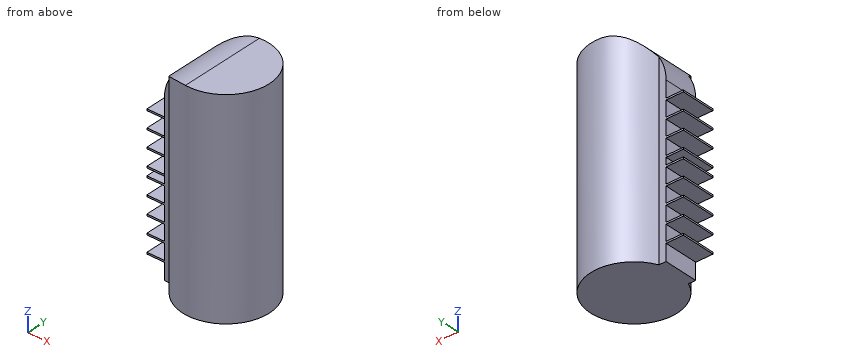
```python
from build123d import *

# Parameters (mm, degrees)
F1_DEPTH = 304.8
F2_R     = 63.5
F4_DEPTH = 25.4


with BuildPart() as f1:
    # F0 (on Top) → F1 (new body)
    with BuildSketch(Plane.XY):
        with BuildLine():
            Line((-68.801289, -25.4), (-58.198711, -25.4))
            ThreePointArc((-58.198711, -25.4), (63.5, 0), (-58.198711, 25.4))
            Line((-58.198711, 25.4), (-68.801289, 25.4))
            Line((-68.801289, 25.4), (-68.801289, -25.4))
        make_face()
    extrude(amount=F1_DEPTH)

    # F2
    f2_edges = [f1.edges().sort_by_distance(p)[0] for p in [
        (-68.801289, 0, 304.8),
    ]]
    fillet(f2_edges, radius=F2_R)

    # F3 (on face) → F4 (join)
    with BuildSketch(Plane(origin=(-68.801289, 0, 0), x_dir=(0, -1, 0), z_dir=(-1, 0, 0))):
        Polygon((-0.093374, 215.9), (-0.093374, 217.17), (-25.4, 217.17), (-25.4, 214.63), (-0.093374, 214.63), align=None)
        Polygon((25.213252, 217.17), (-0.093374, 217.17), (-0.093374, 215.9), (-0.093374, 214.63), (25.213252, 214.63), align=None)
        Polygon((-0.093374, 190.5), (-0.093374, 189.23), (25.213252, 189.23), (25.213252, 191.77), (-0.093374, 191.77), align=None)
        Polygon((-25.4, 191.77), (-25.4, 189.23), (-0.093374, 189.23), (-0.093374, 190.5), (-0.093374, 191.77), align=None)
        Polygon((-25.4, 166.37), (-25.4, 163.83), (-0.093374, 163.83), (-0.093374, 165.1), (-0.093374, 166.37), align=None)
        Polygon((-0.093374, 165.1), (-0.093374, 163.83), (25.213252, 163.83), (25.213252, 166.37), (-0.093374, 166.37), align=None)
        Polygon((-25.4, 128.27), (-25.4, 125.73), (0, 125.73), (0, 127), (-0.009337, 128.27), align=None)
        Polygon((-25.4, 140.97), (-25.4, 138.43), (-0.084037, 138.43), (-0.093374, 139.7), (-0.093374, 140.97), align=None)
        Polygon((-0.093374, 139.7), (-0.084037, 138.43), (25.213252, 138.43), (25.213252, 140.97), (-0.093374, 140.97), align=None)
        Polygon((0, 127), (0, 125.73), (25.4, 125.73), (25.4, 128.27), (-0.009337, 128.27), align=None)
        Polygon((-25.4, 102.87), (-25.4, 100.33), (0, 100.33), (0, 101.6), (0, 102.87), align=None)
        Polygon((0, 101.6), (0, 100.33), (25.4, 100.33), (25.4, 102.87), (0, 102.87), align=None)
        Polygon((-25.4, 77.47), (-25.4, 74.93), (0, 74.93), (0, 76.2), (0, 77.47), align=None)
        Polygon((-25.4, 52.07), (-25.4, 49.53), (0, 49.53), (0, 50.8), (0, 52.07), align=None)
        Polygon((0, 50.8), (0, 49.53), (25.4, 49.53), (25.4, 52.07), (0, 52.07), align=None)
        Polygon((0, 76.2), (0, 74.93), (25.4, 74.93), (25.4, 77.47), (0, 77.47), align=None)
        Polygon((-25.4, 26.67), (-25.4, 24.13), (0, 24.13), (0, 25.4), (0, 26.67), align=None)
        Polygon((0, 25.4), (0, 24.13), (25.4, 24.13), (25.4, 26.67), (0, 26.67), align=None)
    extrude(amount=F4_DEPTH)


solid = f1.part
```
Model file for the job. Use its own axes, mm. Coordinates: 2 decimals unless noted, no trailing zeros. Loops run counter-clockwise (first coordinate to the right, second up) from the corner with the lowest first, then second, coordinate; pieces in that order, holes last. Notation, with made-up numbers: (75, -18.5) - (86, -18.5) arc R25 cw to (86, 8.5) - close; hole circle Ø3 at (33.25, 79.25). An arc over 180 degrees is marked (long way). Write item = value, one per line. Start each with the question number.
Item 1: Saw through at B-B, the plane x = -72. State how many separate pieces and enclosed holes the cut face has, then the cut area to 3 significant figures.
Item 2: Saw through at D-D, the plane x = 30. List the corners of the cut face in (y, z), then the cut area to 3 significant figures.
Item 3: Wall check: probe 1 along X at (y, z) = (-2, 220); probe 2 along Y at (x, z) = (5.5, 190); probe 3 along Y at (x, z) = (2, 208.5). Give the ranges that are in metal, low to high. Write a range as [from, to].
Item 4: Drop flat-ended pins along their axis: pin 1 Ø7.5 at (x, y) = (-80.5, -3) entering from +Z; pin 2 Ø20.5 at (x, y) = (-80.5, 2.5) entering from -Z; pin 3 Ø2 at (x, y) = (-31.5, -37.5) entering from +Z; pin 4 Ø11 at (x, z) = (-80.5, 154) entering from +Y. Give the stop position or say it passes through.
Item 5: Saw through at C-C, the plane z = 153.5. List the corners of the cut face in (x, y), then the cut area to 3 significant figures.
Item 6: Saw through at A-A, the plane y = -50.5. List the corners of the cut face in (x, z).
Answers:
q1.separate_pieces = 9
q1.enclosed_holes = 0
q1.area = 1,160 mm2
q2.outline = (-55.97, 0) - (55.97, 0) - (55.97, 304.8) - (-55.97, 304.8) - close
q2.area = 34,100 mm2
q3.probe_1 = [-68.8, 63.47]
q3.probe_2 = [-63.26, 63.26]
q3.probe_3 = [-63.47, 63.47]
q4.pin_1 = 217.17
q4.pin_2 = 24.13
q4.pin_3 = 299.59
q4.pin_4 = through
q5.outline = (-68.8, -25.4) - (-58.2, -25.4) arc R63.5 ccw (long way) to (-58.2, 25.4) - (-68.8, 25.4) - close
q5.area = 13,000 mm2
q6.outline = (-38.5, 0) - (38.5, 0) - (38.5, 304.8) - (-5.3, 304.8) arc R63.5 ccw to (-38.5, 295.43) - close
